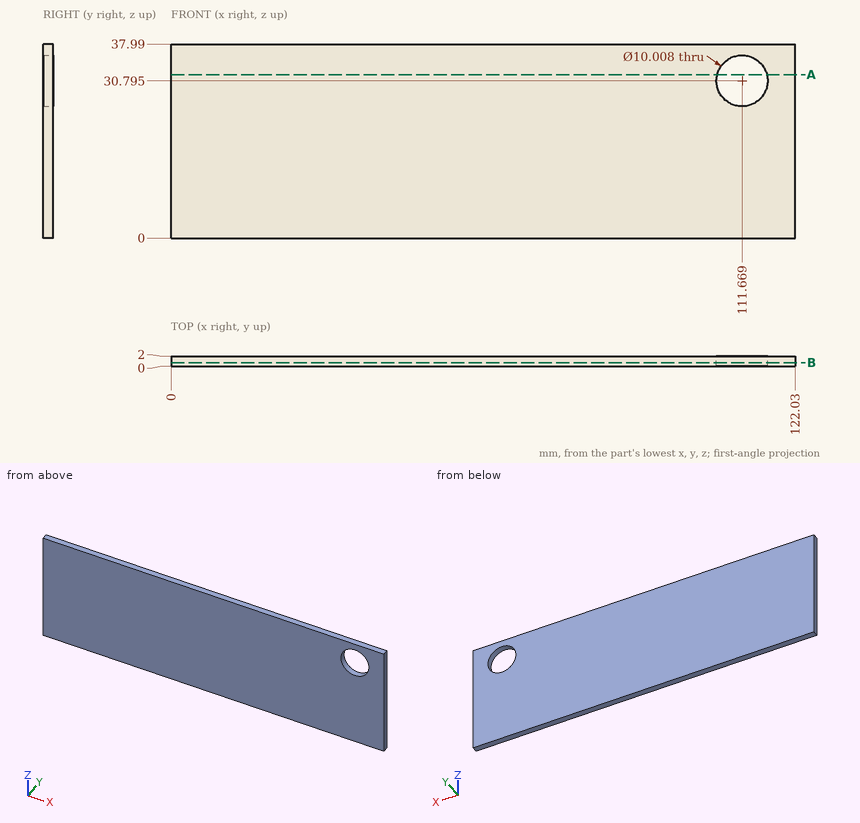
Study the drawing (mm; zero at the part's minimum x, y, z) and answer. Give positions to 0.01 mm unless a question says otherwise; leave off trailing zeros. Write each loop counter-clockwise with the first axis right and the second up, starting at its lowest first coordinate (ties: lowest second). Pieces come first, ordered by that corner, then holes.
Item 1: Find the intervals of material crossed by line 1 along X through (y, z) = (1.8, 28); line 2 along X through (y, z) = (0.4, 32) (1 decimal), in increasing order.
Item 2: Section B-B, the plane y = 0.75 is taken. Write down the section's boundary in (x, z) (1 decimal), plus the area to 3 significant figures.
Item 3: Section A-A, the plane z = 32 is taken. Write down the section's boundary in (x, y) (1 decimal).
Item 4: A flat-ended cylindrical pin translates along its axis: P1, Ø8, axis at x = 111.67, z = 30.8, coming from the -Y side. Find the tip coordinate at first contact, or state that the pin passes through.
Completed:
1. line 1: x = 0 to 107.52, 115.82 to 122.03
1. line 2: x = 0 to 106.8, 116.5 to 122
2. outline: (0, 0) - (122, 0) - (122, 38) - (0, 38) - close; hole circle Ø10 at (111.7, 30.8)
2. area: 4,560 mm2
3. outline: (0, 0) - (106.8, 0) - (106.8, 2) - (0, 2) - close; (116.5, 0) - (122, 0) - (122, 2) - (116.5, 2) - close
4. P1: passes through
